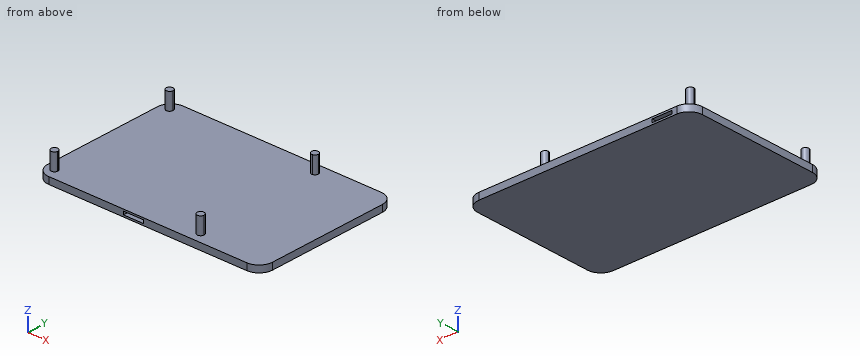
from build123d import *

# Parameters (mm, degrees)
F1_DEPTH = 2.54
F2_R     = 5.08
F3_DEPTH = 8.89
F5_W     = 7.6071470976
F5_H     = 1.2031628285
F6_DEPTH = 4.318
F7_W     = 7.584489882
F7_H     = 1.1869876339
F8_DEPTH = 4.318


# Not quite as in the source:
# - ends of sketch curves that miss each other by under 0.0002 mm in the source are joined


with BuildPart() as f1:
    # F0 (on Top) → F1 (new body)
    with BuildSketch(Plane.XY):
        with BuildLine():
            Line((-42.6210959934, 27.9657971114), (-42.6210959934, 24.0334319246))
            Line((-42.6210959934, 24.0334319246), (-40.4223592815, 24.0334319246))
            ThreePointArc((-40.4223592815, 24.0334319246), (-39.1720464715, 25.4046969243), (-37.8398531152, 24.1128336638))
            ThreePointArc((-37.8398531152, 24.1128336638), (-37.8404635808, 24.0731140337), (-37.8422944012, 24.0334319246))
            Line((-37.8422944012, 24.0334319246), (14.8014883525, 24.0334319246))
            ThreePointArc((14.8014883525, 24.0334319246), (16.1318254594, 25.2445390274), (17.3839117365, 23.9526964724))
            ThreePointArc((17.3839117365, 23.9526964724), (17.080387221, 23.1205499759), (16.312373062, 22.6792460274))
            Line((16.312373062, 22.6792460274), (16.4525141181, -22.7324364705))
            ThreePointArc((16.4525141181, -22.7324364705), (17.3541679288, -23.1175729008), (17.726055436, -24.0247715265))
            ThreePointArc((17.726055436, -24.0247715265), (17.7260481822, -24.0291017499), (17.7260264206, -24.0334319246))
            Line((17.7260264206, -24.0334319246), (42.6210959934, -24.0334319246))
            Line((42.6210959934, -24.0334319246), (42.6210959934, 24.0334319246))
            Line((42.6210959934, 24.0334319246), (42.6210959934, 27.965891646))
            Line((42.6210959934, 27.965891646), (-42.6210959934, 27.9657971114))
        make_face()
        with BuildLine():
            Line((-42.6210959934, 24.0334319246), (-42.6210959934, -24.0334319246))
            Line((-42.6210959934, -24.0334319246), (-40.4303500829, -24.0334319246))
            ThreePointArc((-40.4303500829, -24.0334319246), (-39.2142367954, -22.6050090303), (-37.8527686966, -23.8956399262))
            ThreePointArc((-37.8527686966, -23.8956399262), (-37.8546115269, -23.9646342987), (-37.8601347627, -24.0334319246))
            Line((-37.8601347627, -24.0334319246), (15.1411369991, -24.0334319246))
            ThreePointArc((15.1411369991, -24.0334319246), (15.5233039011, -23.1072298959), (16.4525141181, -22.7324364705))
            Line((16.4525141181, -22.7324364705), (16.312373062, 22.6792460274))
            ThreePointArc((16.312373062, 22.6792460274), (15.2287950262, 22.9902332706), (14.8014883525, 24.0334319246))
            Line((14.8014883525, 24.0334319246), (-37.8422944012, 24.0334319246))
            ThreePointArc((-37.8422944012, 24.0334319246), (-39.1323268414, 22.8203599376), (-40.4223592815, 24.0334319246))
            Line((-40.4223592815, 24.0334319246), (-42.6210959934, 24.0334319246))
        make_face()
        with BuildLine():
            Line((-40.4303500829, -24.0334319246), (-42.6210959934, -24.0334319246))
            Line((-42.6210959934, -24.0334319246), (-42.6210959934, -27.965891646))
            Line((-42.6210959934, -27.965891646), (42.6210959934, -27.965891646))
            Line((42.6210959934, -27.965891646), (42.6210959934, -24.0334319246))
            Line((42.6210959934, -24.0334319246), (17.7260264206, -24.0334319246))
            ThreePointArc((17.7260264206, -24.0334319246), (16.4335817099, -25.3172452526), (15.1411369991, -24.0334319246))
            Line((15.1411369991, -24.0334319246), (-37.8601347627, -24.0334319246))
            ThreePointArc((-37.8601347627, -24.0334319246), (-39.1452424228, -25.1881136524), (-40.4303500829, -24.0334319246))
        make_face()
    extrude(amount=F1_DEPTH)

    # F2
    f2_edges = [f1.edges().sort_by_distance(p)[0] for p in [
        (42.621096, -27.965892, 1.27),
        (-42.621096, -27.965892, 1.27),
        (42.621096, 27.965892, 1.27),
        (-42.621096, 27.965797, 1.27),
    ]]
    fillet(f2_edges, radius=F2_R)

    # F0 (on Top) → F3 (join)
    with BuildSketch(Plane.XY):
        with BuildLine():
            ThreePointArc((-37.8398531152, 24.1128336638), (-39.1720464715, 25.4046969243), (-40.4223592815, 24.0334319246))
            Line((-40.4223592815, 24.0334319246), (-37.8422944012, 24.0334319246))
            ThreePointArc((-37.8422944012, 24.0334319246), (-37.8404635808, 24.0731140337), (-37.8398531152, 24.1128336638))
        make_face()
        with BuildLine():
            Line((-37.8422944012, 24.0334319246), (-40.4223592815, 24.0334319246))
            ThreePointArc((-40.4223592815, 24.0334319246), (-39.1323268414, 22.8203599376), (-37.8422944012, 24.0334319246))
        make_face()
        with BuildLine():
            ThreePointArc((-37.8527686966, -23.8956399262), (-39.2142367954, -22.6050090303), (-40.4303500829, -24.0334319246))
            Line((-40.4303500829, -24.0334319246), (-37.8601347627, -24.0334319246))
            ThreePointArc((-37.8601347627, -24.0334319246), (-37.8546115269, -23.9646342987), (-37.8527686966, -23.8956399262))
        make_face()
        with BuildLine():
            Line((-37.8601347627, -24.0334319246), (-40.4303500829, -24.0334319246))
            ThreePointArc((-40.4303500829, -24.0334319246), (-39.1452424228, -25.1881136524), (-37.8601347627, -24.0334319246))
        make_face()
        with BuildLine():
            ThreePointArc((17.3839117365, 23.9526964724), (16.1318254594, 25.2445390274), (14.8014883525, 24.0334319246))
            Line((14.8014883525, 24.0334319246), (16.3081940264, 24.0334319246))
            Line((16.3081940264, 24.0334319246), (16.312373062, 22.6792460274))
            ThreePointArc((16.312373062, 22.6792460274), (17.080387221, 23.1205499759), (17.3839117365, 23.9526964724))
        make_face()
        with BuildLine():
            Line((16.3081940264, 24.0334319246), (14.8014883525, 24.0334319246))
            ThreePointArc((14.8014883525, 24.0334319246), (15.2287950262, 22.9902332706), (16.312373062, 22.6792460274))
            Line((16.312373062, 22.6792460274), (16.3081940264, 24.0334319246))
        make_face()
        with BuildLine():
            Line((16.4525141181, -22.7324364705), (16.4565290074, -24.0334319246))
            Line((16.4565290074, -24.0334319246), (17.7260264206, -24.0334319246))
            ThreePointArc((17.7260264206, -24.0334319246), (17.7260481822, -24.0291017499), (17.726055436, -24.0247715265))
            ThreePointArc((17.726055436, -24.0247715265), (17.3541679288, -23.1175729008), (16.4525141181, -22.7324364705))
        make_face()
        with BuildLine():
            ThreePointArc((16.4525141181, -22.7324364705), (15.5233039011, -23.1072298959), (15.1411369991, -24.0334319246))
            Line((15.1411369991, -24.0334319246), (16.4565290074, -24.0334319246))
            Line((16.4565290074, -24.0334319246), (16.4525141181, -22.7324364705))
        make_face()
        with BuildLine():
            Line((16.4565290074, -24.0334319246), (15.1411369991, -24.0334319246))
            ThreePointArc((15.1411369991, -24.0334319246), (16.4335817099, -25.3172452526), (17.7260264206, -24.0334319246))
            Line((17.7260264206, -24.0334319246), (16.4565290074, -24.0334319246))
        make_face()
    extrude(amount=F3_DEPTH)

    # F5 (on face) → F6 (cut)
    with BuildSketch(Plane.XZ.offset(27.965891646)):
        with Locations((-5.5109024979, 1.2853431981)):
            Rectangle(F5_W, F5_H)
    extrude(amount=-F6_DEPTH, mode=Mode.SUBTRACT)

    # F7 (on face) → F8 (cut)
    with BuildSketch(Plane(origin=(0, 27.965891646, 0), x_dir=(-1, 0, 0), z_dir=(0, 1, 0))):
        with Locations((31.9627784193, 1.27)):
            Rectangle(F7_W, F7_H)
    extrude(amount=-F8_DEPTH, mode=Mode.SUBTRACT)


solid = f1.part
Here's how the part is built. I have some questions about the finished solid (model axes, mm). Round coordinates to 2 decimals unless told otherwise and drop trailing zeros. Write each loop counter-clockwise with the first axis right and the second up, starting at its lowest first coordinate (ties: lowest second). Pieces come first, ordered by that corner, then holes.
1. Suppose I cut it at C-C (x = -13.5). List the corners of the cut face in (y, z) for me, and give its area (3 significant figures).
2. Suppose I cut it at B-B (y = 3). List the corners of the cut face in (x, z) for me, and give its area (3 significant figures).
3. Will these pins go through, and if not, where does the flat tip stop? pin 1 Ø0.6 at (y, z) = (25, 1.5) entering from -X; pin 2 Ø12 at (x, y) = (5, 18) entering from +Z; pin 3 Ø0.9 at (y, z) = (26.5, 1.5) entering from +X.
4. I need wall thicknesses on L1, parallel to Z at x = 15, y = -11.5; L2, parallel to X at y = 23.5, z = 5; L3, parallel to X at y = 24.5, z = 3.75. Which ranges of each line are inside material? Lowest first, please.
5. Suppose I cut it at A-A (z = 7.5). State how many separate pieces and enclosed holes the cut face has, and give its area (3 significant figures).
Answer sheet:
1. outline: (-27.97, 0) - (27.97, 0) - (27.97, 2.54) - (-27.97, 2.54) - close
1. area: 142 mm2
2. outline: (-42.62, 0) - (42.62, 0) - (42.62, 2.54) - (-42.62, 2.54) - close
2. area: 217 mm2
3. pin 1: stops at x = -42.29
3. pin 2: stops at z = 2.54
3. pin 3: stops at x = 41.52
4. L1: z = 0 to 2.54
4. L2: x = -40.27 to -37.99, 14.88 to 17.3
4. L3: x = -40.37 to -37.9, 14.92 to 17.26
5. separate pieces: 4
5. enclosed holes: 0
5. area: 21.0 mm2
